Geometry check sheet. Reference: the model listing, model coordinates, mm. Face numbers are marked on the shaded views. A direction names the side the tool comes from. Coordinates: 2 decimals unless noted, no trailing zeros. Write each loop counter-clockwise with the first axis right and the second up, starting at its lowest first coordinate (ties: lowest second). Pieces come first, ordered by that corner, then holes. Notation, with made-up numbers: (50.25, -12.75) -> (93.25, -12.75) arc R12 ccw to (93.25, 10.25) -> close; hole circle Ø10 at (52, 26.25). An arc over 180 degrees is marked (long way). One line per question, with ' | ' between items.
Autodesk Inventor part; units mm, degrees
ref_plane "YZ Plane" through (0, 0, 0) normal (1, 0, 0) x (0, 1, 0)
ref_plane "XZ Plane" through (0, 0, 0) normal (0, 1, 0) x (-1, 0, 0)
ref_plane "XY Plane" through (0, 0, 0) normal (0, 0, 1) x (1, 0, 0)
sketch "Sketch1" plane through (0, 0, 0) normal (0, 1, 0) x (-1, 0, 0)
  line L0 (0, 0) -> (152.4, 0)
  line L1 (152.4, 0) -> (152.4, 50.8)
  line L2 (152.4, 50.8) -> (0, 50.8)
  line L3 (0, 50.8) -> (0, 0)
  dimension "d0" = 152.4
  dimension "d1" = 50.8
extrude "Extrusion1" add sketch "Sketch1" along normal blind 5.08
sketch "Sketch2" plane through (0, 5.08, 0) normal (0, 1, 0) x (1, 0, 0)
  line L0 (0, 0) -> (-152.4, 0)
  line L1 (-152.4, -50.8) -> (0, -50.8)
  line L2 (-76.2, 0) -> (-76.2, -25.4)
  line L3 (-76.2, -25.4) -> (-59.69, -25.4)
  line L4 (-59.69, -25.4) -> (-59.69, -8.89)
  line L5 (-59.69, -8.89) -> (-53.34, -8.89)
  line L6 (-53.34, -8.89) -> (-53.34, -50.8)
  line L7 (-53.34, -8.89) -> (-53.34, 0)
  line L8 (-53.34, 0) -> (-50.8, 0)
  line L9 (-50.8, 0) -> (-50.8, -50.8)
  line L10 (-53.34, -50.8) -> (-50.8, -50.8)
  dimension "d4" = 16.51
  dimension "d5" = 16.51
  dimension "d6" = 6.35
  dimension "d7" = 2.54
extrude "Extrusion2" add sketch "Sketch2" along normal blind 36.83 contours L9 L1 L6 L7 L0
sketch "Sketch3" plane through (0, 5.08, 0) normal (0, 1, 0) x (1, 0, 0)
  line L0 (-53.34, 0) -> (-152.4, 0)
  line L1 (-152.4, -50.8) -> (-53.34, -50.8)
  line L2 (-152.4, 0) -> (-76.2, 0)
  line L3 (-76.2, 0) -> (-76.2, -25.4)
  line L4 (-76.2, -25.4) -> (-92.71, -25.4)
  line L5 (-92.71, -25.4) -> (-99.06, -25.4)
  line L6 (-99.06, -25.4) -> (-99.06, 0)
  line L7 (-99.06, 0) -> (-101.6, 0)
  line L8 (-101.6, 0) -> (-101.6, -50.8)
  line L9 (-101.6, -50.8) -> (-99.06, -50.8)
  line L10 (-99.06, -25.4) -> (-99.06, -50.8)
  point P0 (0, 0)
  dimension "d10" = 76.2
  dimension "d11" = 16.51
  dimension "d12" = 6.35
  dimension "d13" = 2.54
extrude "Extrusion3" add sketch "Sketch3" along normal blind 36.83 contours L6 L10 L1 L8 L0
sketch "Sketch4" plane through (0, 41.91, 0) normal (0, 1, 0) x (1, 0, 0)
  line L0 (-101.6, 0) -> (-101.6, -50.8)
  line L1 (-101.6, 0) -> (-50.8, 0)
  line L2 (-50.8, 0) -> (-50.8, -50.8)
  line L3 (-50.8, -50.8) -> (-101.6, -50.8)
  point P0 (0, 0)
  dimension "d16" = 50.8
extrude "Extrusion4" add sketch "Sketch4" along normal blind 2.54
sketch "Sketch5" plane through (0, 5.08, 0) normal (0, 1, 0) x (1, 0, 0)
  line L0 (-99.06, 0) -> (-99.06, -50.8)
  line L1 (-99.06, -50.8) -> (-53.34, -50.8)
  line L2 (-53.34, -50.8) -> (-53.34, 0)
  line L3 (-53.34, 0) -> (-99.06, 0)
  point P0 (0, 0)
extrude "Extrusion5" cut sketch "Sketch5" against normal blind 13.6525
sketch "Sketch6" plane through (0, 44.45, 0) normal (0, 1, 0) x (1, 0, 0)
  line L0 (-50.8, 0) -> (-101.6, 0)
  line L1 (-101.6, 0) -> (-101.6, -50.8)
  line L2 (-76.2, 0) -> (-76.2, -25.4)
  circle A0 centre (-76.2, -25.4) radius 12.7
  line L3 (-76.2, -25.4) -> (-59.69, -25.4)
  line L4 (-59.69, -25.4) -> (-59.69, -8.89)
  circle A1 centre (-59.69, -8.89) radius 2.54
  line L5 (-59.69, -25.4) -> (-59.69, -41.91)
  circle A2 centre (-59.69, -41.91) radius 2.54
  line L6 (-76.2, -25.4) -> (-92.71, -25.4)
  line L7 (-92.71, -25.4) -> (-92.71, -8.89)
  circle A3 centre (-92.71, -8.89) radius 2.54
  line L8 (-92.71, -25.4) -> (-92.71, -41.91)
  circle A4 centre (-92.71, -41.91) radius 2.54
  point P0 (0, 0)
  dimension "d21" = 25.4
  dimension "d22" = 16.51
  dimension "d23" = 16.51
  dimension "d24" = 5.08
  dimension "d25" = 16.51
  dimension "d26" = 5.08
  dimension "d27" = 16.51
  dimension "d28" = 16.51
  dimension "d29" = 5.08
  dimension "d30" = 16.51
  dimension "d31" = 5.08
extrude "Extrusion6" cut sketch "Sketch6" against normal blind 13.6525
sketch "Sketch7" plane through (0, 5.08, 0) normal (0, 1, 0) x (1, 0, 0)
  line L0 (0, -50.8) -> (0, 0)
  line L1 (0, 0) -> (-50.8, 0)
  line L2 (0, 0) -> (25.4, 0)
  line L3 (25.4, 0) -> (25.4, -50.8)
  line L4 (25.4, -50.8) -> (0, -50.8)
  dimension "d34" = 25.4
extrude "Extrusion7" add sketch "Sketch7" against normal blind 5.08
sketch "Sketch8" plane through (-152.4, 0, 0) normal (-1, 0, 0) x (0, 0, 1)
  line L0 (0, 0) -> (50.8, 0)
  line L1 (50.8, 0) -> (50.8, 5.08)
  line L2 (0, 5.08) -> (50.8, 5.08)
  line L3 (0, 0) -> (0, 5.08)
extrude "Extrusion8" add sketch "Sketch8" along normal blind 25.4
sketch "Sketch9" plane through (0, 5.08, 0) normal (0, 1, 0) x (1, 0, 0)
  line L0 (-101.6, 0) -> (-177.8, 0)
  line L1 (-101.6, 0) -> (-152.4, 0)
  line L2 (-152.4, 0) -> (-152.4, -25.4)
  circle A0 centre (-152.4, -25.4) radius 6
  circle A1 centre (-152.4, -25.4) radius 3
  point P0 (0, 0)
  dimension "d39" = 50.8
  dimension "d40" = 12
  dimension "d41" = 6
extrude "Extrusion9" add sketch "Sketch9" along normal blind 19.05
sketch "Sketch10" plane through (0, 5.08, 0) normal (0, 1, 0) x (1, 0, 0)
  line L0 (25.4, 0) -> (-50.8, 0)
  line L1 (-50.8, 0) -> (0, 0)
  line L2 (0, 0) -> (0, -25.4)
  line L3 (0, -25.4) -> (0, 0)
  circle A0 centre (0, -25.4) radius 3
  circle A1 centre (0, -25.4) radius 6
  dimension "d44" = 50.8
  dimension "d45" = 6
  dimension "d46" = 12
extrude "Extrusion10" add sketch "Sketch10" along normal blind 19.05
fillet "Fillet1" radius 4.7625 2 edges at (-158.4, 5.08, 25.4) (-6, 5.08, 25.4)
fillet "Fillet2" radius 20.6375 2 edges at (-50.8, 5.08, 25.4) (-101.6, 5.08, 25.4)
sketch "Sketch11" plane through (0, 5.08, 0) normal (0, 1, 0) x (1, 0, 0)
  line L0 (-122.2375, 0) -> (-177.8, 0)
  line L1 (-122.2375, -50.8) -> (-177.8, -50.8)
  line L2 (-177.8, 0) -> (-165.1, 0)
  line L3 (-165.1, 0) -> (-165.1, -12.7)
  circle A0 centre (-165.1, -12.7) radius 3.175
  line L4 (-177.8, -50.8) -> (-165.1, -50.8)
  line L5 (-165.1, -50.8) -> (-165.1, -38.1)
  circle A1 centre (-165.1, -38.1) radius 3.175
  point P0 (0, 0)
  dimension "d51" = 12.7
  dimension "d52" = 12.7
  dimension "d53" = 6.35
  dimension "d54" = 12.7
  dimension "d55" = 12.7
  dimension "d56" = 6.35
extrude "Extrusion11" cut sketch "Sketch11" against normal blind 19.05
sketch "Sketch12" plane through (0, 5.08, 0) normal (0, 1, 0) x (1, 0, 0)
  line L0 (-30.1625, -50.8) -> (25.4, -50.8)
  line L1 (25.4, 0) -> (-30.1625, 0)
  line L2 (25.4, 0) -> (12.7, 0)
  line L3 (12.7, 0) -> (12.7, -12.7)
  circle A0 centre (12.7, -12.7) radius 3.175
  line L4 (25.4, -50.8) -> (12.7, -50.8)
  line L5 (12.7, -50.8) -> (12.7, -38.1)
  circle A1 centre (12.7, -38.1) radius 3.175
  point P0 (0, 0)
  dimension "d59" = 12.7
  dimension "d60" = 12.7
  dimension "d61" = 6.35
  dimension "d62" = 12.7
  dimension "d63" = 12.7
  dimension "d64" = 6.35
extrude "Extrusion12" cut sketch "Sketch12" against normal blind 19.05
sketch "Sketch13" plane through (0, 5.08, 0) normal (0, 1, 0) x (1, 0, 0)
  line L0 (-122.2375, 0) -> (-177.8, 0)
  line L1 (-177.8, 0) -> (-133.35, 0)
  line L2 (-133.35, 0) -> (-133.35, -25.4)
  circle A0 centre (-133.35, -25.4) radius 4.445
  point P0 (0, 0)
  dimension "d67" = 44.45
  dimension "d68" = 8.89
sketch "Sketch14" plane through (0, 5.08, 0) normal (0, 1, 0) x (1, 0, 0)
  line L0 (25.4, 0) -> (-30.1625, 0)
  line L1 (25.4, 0) -> (-19.05, 0)
  line L2 (-19.05, 0) -> (-19.05, -25.4)
  circle A0 centre (-19.05, -25.4) radius 4.445
  point P0 (0, 0)
  dimension "d69" = 44.45
  dimension "d70" = 8.89
extrude "Extrusion13" cut sketch "Sketch13" against normal blind 19.05
extrude "Extrusion14" cut sketch "Sketch14" against normal blind 19.05
sketch "Sketch15" plane through (0, 44.45, 0) normal (0, 1, 0) x (1, 0, 0)
  circle A0 centre (-92.71, -41.91) radius 2.54
  circle A1 centre (-59.69, -41.91) radius 2.54
  circle A2 centre (-59.69, -8.89) radius 2.54
  circle A3 centre (-92.71, -8.89) radius 2.54
  circle A4 centre (-76.2, -25.4) radius 12.7
  line L0 (-101.6, -50.8) -> (-50.8, -50.8)
  line L1 (-50.8, -50.8) -> (-50.8, 0)
  line L2 (-50.8, 0) -> (-101.6, 0)
  line L3 (-101.6, 0) -> (-101.6, -50.8)
  point P0 (0, 0)
properties part number "Base plate"
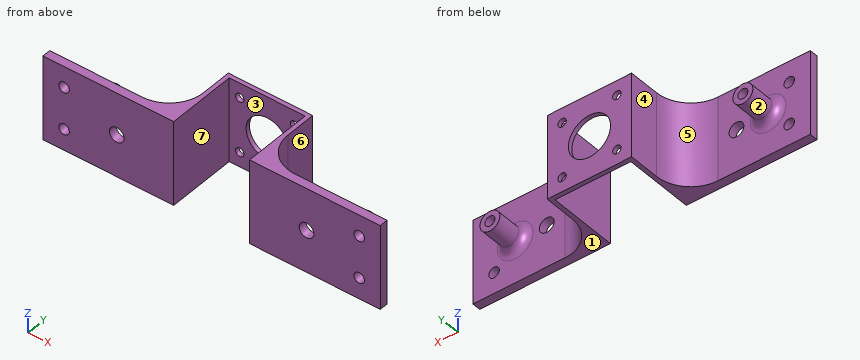
1. Go/stop test with flat-tipped pins: P1, Ø4, axis at y = 25.5, z = 6, coming from the -X side; P2, Ø15, axis at y = 37.5, z = 34.5, coming from the -X side; P3, Ø1.5, axis at y = 34, z = 6.5, coming from the +X side; P4, Ø5.5, axis at x = -165.1, z = 12.7, coming from the +Y side. Record where each tip stops, or that it passes through.
Worked answers:
P1: x = -101.72 | P2: x = -101.6 | P3: x = -50.8 | P4: through
2. Mould release check, pull along X, two halves, no side actions. Record for the marked faces 1, 2, 3 and 4: released by +X, released by -X, zero draft, split by the parting line, or undercut.
Worked answers:
face 1: zero draft | face 2: undercut | face 3: undercut | face 4: released by -X
3. Cross-section at B-B on y = 3. Record the boundary of the cut face in (x, z) (3 decimals).
Worked answers:
outline: (-177.8, 0) -> (-99.06, 0) -> (-99.06, 50.8) -> (-177.8, 50.8) -> close; (-53.34, 0) -> (25.4, 0) -> (25.4, 50.8) -> (-53.34, 50.8) -> close; hole circle Ø6.35 at (-165.1, 12.7); hole circle Ø6.35 at (-165.1, 38.1); hole circle Ø8.89 at (-133.35, 25.4); hole circle Ø8.89 at (-19.05, 25.4); hole circle Ø6.35 at (12.7, 12.7); hole circle Ø6.35 at (12.7, 38.1)
4. Cross-section at A-A on x = -59.69. Record the boundary of the cut face in (y, z), and give its area (3 significant figures).
Worked answers:
outline: (41.91, 0) -> (44.45, 0) -> (44.45, 6.35) -> (41.91, 6.35) -> close; (41.91, 11.43) -> (44.45, 11.43) -> (44.45, 39.37) -> (41.91, 39.37) -> close; (41.91, 44.45) -> (44.45, 44.45) -> (44.45, 50.8) -> (41.91, 50.8) -> close | area: 103 mm²
5. Cross-section at C-C on y = 34. Record the boundary of the cut face in (x, z), and give its area (3 significant figures).
Worked answers:
outline: (-101.6, 0) -> (-99.06, 0) -> (-99.06, 50.8) -> (-101.6, 50.8) -> close; (-53.34, 0) -> (-50.8, 0) -> (-50.8, 50.8) -> (-53.34, 50.8) -> close | area: 258 mm²
6. Material ranges on line 1 (X direction, y = 42.6, z = 8.89); line 2 (X direction, y = 3.5, z = 42.5); line 3 (X direction, y = 24.5, z = 12), recorded low to high. Write a range as from..to.
Worked answers:
line 1: -101.6..-95.25, -90.17..-62.23, -57.15..-50.8 | line 2: -177.8..-99.06, -53.34..25.4 | line 3: -101.64..-99.06, -53.34..-50.76
7. Tool access check on the marked faces 5, 6 and 7. Record the directions out of +Z, -Z, +X, -X, +Y, -Y that give a thin tool (end or side, any length) a straight path to the whole face; none if there is none.
Worked answers:
face 5: +Z, -Z, +Y | face 6: +Z, -Z, +X, +Y | face 7: +Z, -Z, -Y
8. Cross-section at D-D on x = 0. Record the boundary of the cut face in (y, z) (1 decimal), and give its area (3 significant figures).
Worked answers:
outline: (0, 0) -> (5.1, 0) -> (5.1, 14.6) arc R4.8 cw to (9.8, 19.4) -> (24.1, 19.4) -> (24.1, 22.4) -> (5.1, 22.4) -> (5.1, 28.4) -> (24.1, 28.4) -> (24.1, 31.4) -> (9.8, 31.4) arc R4.8 cw to (5.1, 36.2) -> (5.1, 50.8) -> (0, 50.8) -> close | area: 382 mm²
